Read the model definition and answer for the solid it produces. Units are mm, in the model's axes. A direction names the side the tool comes from. Give positions to 0.01 mm unless a question says otherwise; leave off trailing zeros. Order: outer loops, then holes, each group sorted by start corner. A loop starts at its lowest first (then second) coordinate and runs counter-clockwise, first axis right, second up. Notation, with made-up numbers: M 15.25,10 L 36.25,10 A29 ccw 36.25,43 Z; hole C -22,53.5 d5. An arc over 180 degrees is marked long. One line per item, written item: value.
from build123d import *

# Parameters (mm, degrees)
BOSS_EXTRUDE1_DEPTH = 10
SKETCH1_3_W         = 7.5
SKETCH1_3_H         = 28.942025954
BOSS_EXTRUDE2_DEPTH = 5
SKETCH1_4_W         = 30
SKETCH1_4_H         = 2.807974046
BOSS_EXTRUDE3_DEPTH = 20
SKETCH2_R           = 2
CUT_EXTRUDE1_DEPTH  = 20


with BuildPart() as part:
    # Sketch1 → Boss-Extrude1 (new body)
    with BuildSketch(Plane.XY):
        Polygon((6.5, 5.25), (6.5, 0), (7.5, 0), (7.5, -8.25), (9.5, -8.25), (9.5, 8.25), (-9.5, 8.25), (-9.5, -8.25), (-7.5, -8.25), (-7.5, 0), (-6.5, 0), (-6.5, 5.25), align=None)
        Polygon((0, -8.25), (0, -5.25), (-6.5, -5.25), (-6.5, 0), (-7.5, 0), (-7.5, -8.25), align=None)
        Polygon((6.5, -5.25), (0, -5.25), (0, -8.25), (7.5, -8.25), (7.5, 0), (6.5, 0), align=None)
    extrude(amount=BOSS_EXTRUDE1_DEPTH)

    # Sketch1_3 → Boss-Extrude2 (add)
    with BuildSketch(Plane.XY):
        with Locations((-3.75, -22.721012977)):
            Rectangle(SKETCH1_3_W, SKETCH1_3_H)
        with Locations((3.75, -22.721012977)):
            Rectangle(SKETCH1_3_W, SKETCH1_3_H)
    extrude(amount=BOSS_EXTRUDE2_DEPTH)

    # Sketch1_4 → Boss-Extrude3 (add)
    with BuildSketch(Plane.XY):
        with Locations((0, -38.596012977)):
            Rectangle(SKETCH1_4_W, SKETCH1_4_H)
    extrude(amount=BOSS_EXTRUDE3_DEPTH)

    # Sketch2 → Cut-Extrude1 (cut)
    with BuildSketch(Plane(origin=(0, -37.192025954, 0), x_dir=(1, 0, 0), z_dir=(0, 1, 0))):
        with Locations(Location((-10, -15, 0), (0, 0, 270))):
            Circle(SKETCH2_R)
        with Locations(Location((10, -15, 0), (0, 0, 270))):
            Circle(SKETCH2_R)
    extrude(amount=-CUT_EXTRUDE1_DEPTH, mode=Mode.SUBTRACT)


solid = part.part
1) Find section D-D, the plane y = 4.5. Write down the section's boundary in (x, z).
Reported:
outline: M -9.5,0 L -6.5,0 L -6.5,10 L -9.5,10 Z; M 6.5,0 L 9.5,0 L 9.5,10 L 6.5,10 Z
2) Find section C-C, the plane z = 15. Write down the section's boundary in (x, y), plus the area to 3 significant figures.
Reported:
outline: M -15,-40 L -12,-40 L -12,-37.19 L -15,-37.19 Z; M -8,-40 L 8,-40 L 8,-37.19 L -8,-37.19 Z; M 12,-40 L 15,-40 L 15,-37.19 L 12,-37.19 Z
area: 61.8 mm^2
3) Each of these flat-tipped pins is pushed along its axis until it touches: pin 1 Ø3 at (x, z) = (10, 15) entering from -Y; pin 2 Ø8 at (y, z) = (-2, 5.5) entering from +X; pin 3 Ø7.5 at (x, y) = (3, -29) entering from +Z; pin 4 Ø8 at (y, z) = (1, 3.5) entering from -X. Where does it stop, or does it pass through?
Reported:
pin 1: passes through
pin 2: stops at x = 9.5
pin 3: stops at z = 5
pin 4: stops at x = -9.5
4) Find section B-B, the plane x = -3. Write down the section's boundary in (y, z).
Reported:
outline: M -40,0 L -5.25,0 L -5.25,10 L -8.25,10 L -8.25,5 L -37.19,5 L -37.19,20 L -40,20 Z; M 5.25,0 L 8.25,0 L 8.25,10 L 5.25,10 Z
5) Determine the mould class of faces 1 (the face through (15, -39, 10)), 2 (the face through (-6.5, 0, 5)), 3 (the face through (0, -40, 10)) for opening direction Y: +Y half, -Y half, draft (parallel to the pull), parting line (faces both ways), or undercut.
Reported:
face 1: draft
face 2: undercut
face 3: -Y half
6) Consider probe 1 along Y at (x, z) = (1, 7.25); probe 2 along X at (y, z) = (-38, 15); probe 3 along Y at (x, z) = (8.25, 8.5). Determine where each line is inside the solid, lowest interval first.
Reported:
probe 1: y = -40 to -37.19, -8.25 to -5.25, 5.25 to 8.25
probe 2: x = -15 to -12, -8 to 8, 12 to 15
probe 3: y = -40 to -37.19, -8.25 to 8.25
7) Find section A-A, the plane z = 5.5. Write down the section's boundary in (x, y).
Reported:
outline: M -15,-40 L 15,-40 L 15,-37.19 L -15,-37.19 Z; M -9.5,-8.25 L 9.5,-8.25 L 9.5,8.25 L -9.5,8.25 Z; hole M -6.5,-5.25 L 6.5,-5.25 L 6.5,5.25 L -6.5,5.25 Z
8) Which of the six approach directions +Z, -Z, +X, -X, +Y, -Y give full straight-line access (tool end or side, diameter ignored) to faces 4 (the face through (-7.5, -23, 2)), 5 (the face through (-9.5, 0, 5)), 6 (the face through (0, 6, 10))?
Reported:
face 4: +Z, -Z, -X
face 5: +Z, -Z, -X, +Y
face 6: +Z, +X, -X, +Y
